Input: part model. Units: mm. Frame: model coordinates. A direction names the side the tool comes from. Round coordinates to 2 decimals unless told otherwise and drop trailing zeros. Order: outer loops, then holes, each group sorted by start corner. A loop starts at its lowest first (then second) coordinate and runs counter-clockwise, first axis right, second up. Notation, with made-up numbers: (-4, 29.25) - (1, 29.25) arc R15 cw to (1, 40.25) - close; hole circle Ø3 at (47.5, 60). An arc over 180 degrees is marked (long way). One line per item, written item: value. Start each with the question number.
from build123d import *

# Parameters (mm, degrees)
F4_DEPTH = 10


with BuildPart() as f1:
    # F0 (on Front) → F1 (revolve)
    with BuildSketch(Plane.XZ):
        Polygon((-500, 37.5), (-500, 0), (500, 0), (500, 37.5), (400, 37.5), (400, 50), (-400, 50), (-400, 37.5), align=None)
    revolve(axis=Axis((0, 0, 0), (1, 0, 0)))

    # F3 (on offset) → F4 (cut)
    with BuildSketch(Plane.XY.offset(37.5)):
        with BuildLine():
            Line((-450, 10), (-500, 10))
            Line((-500, 10), (-500, -10))
            Line((-500, -10), (-450, -10))
            ThreePointArc((-450, -10), (-440, 0), (-450, 10))
        make_face()
        with BuildLine():
            ThreePointArc((450, 10), (440, 0), (450, -10))
            Line((450, -10), (500, -10))
            Line((500, -10), (500, 10))
            Line((500, 10), (450, 10))
        make_face()
    extrude(amount=-F4_DEPTH, mode=Mode.SUBTRACT)


solid = f1.part
1. Section B-B (y = 0). Return the cut outline in (x, z), then the cut area to 3 significant figures.
2. Line query: line 1 (X direction, y = 30.5, z = 33); line 2 (Z direction, x = 4, y = -2); line 3 (Y direction, x = -447, z = -15.5). Output: solid intervals per line, ascending. Write a range as from..to.
3. Section C-C (x = -80.5). Return the cut outline in (y, z).
4. Pull-direction query (Y, two-part tool) for faces 6 (the face through (-500, -1, -1)), 7 (the face through (-450.7, -37.18, -4.88)), 8 (the face through (470, 0, 27.5)); classes: released by +Y, released by -Y, zero draft, split by the parting line, or undercut.
5. Section A-A (z = 0). Return the cut outline in (x, y).
6. Set-up query: faces 1 (the face through (500, -1, 0)), 2 (the face through (449.3, -37.18, -4.88)), 3 (the face through (-400, -37, 7)), 4 (the face through (-5.6, -15.02, 47.69)), 5 (the face through (-470, 0, 27.5)). Return all of +Z, -Z, +X, -X, +Y, -Y with unobstructed straight access to the full face (end or side cutting, diameter ignored); none if empty.
7. Pin query (flat end, axial travel): pin 1 (3 mm diameter, centred on x = -390, z = 31, fed in from +Y); pin 2 (9.5 mm diameter, centred on x = -470.5, z = 32, fed in from +Y); pin 3 (12 mm diameter, centred on x = 278.5, z = -33, fed in from -Y). Return the tip coordinate at first contact, or that it passes through.
Solved:
1. outline: (-500, -37.5) - (-400, -37.5) - (-400, -50) - (400, -50) - (400, -37.5) - (500, -37.5) - (500, 27.5) - (440, 27.5) - (440, 37.5) - (400, 37.5) - (400, 50) - (-400, 50) - (-400, 37.5) - (-440, 37.5) - (-440, 27.5) - (-500, 27.5) - close
1. area: 93,800 mm²
2. line 1: x = -400..400
2. line 2: z = -49.96..49.96
2. line 3: y = -34.15..34.15
3. outline: circle Ø100 at (0, 0)
4. face 6: zero draft
4. face 7: split by the parting line
4. face 8: undercut
5. outline: (-500, -37.5) - (-400, -37.5) - (-400, -50) - (400, -50) - (400, -37.5) - (500, -37.5) - (500, 37.5) - (400, 37.5) - (400, 50) - (-400, 50) - (-400, 37.5) - (-500, 37.5) - close
6. face 1: +Z, -Z, +X, +Y, -Y
6. face 2: +X
6. face 3: -X
6. face 4: +X, -X
6. face 5: +Z, -X
7. pin 1: stops at y = 40.37
7. pin 2: stops at y = 25.76
7. pin 3: stops at y = -42.08
